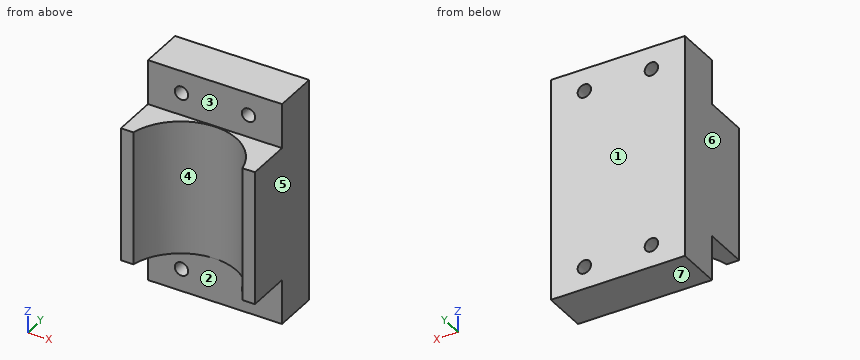
from build123d import *

# Parameters (mm, degrees)
F0_W     = 30
F0_H     = 50
F1_DEPTH = 10
F2_R     = 1.5
F3_DEPTH = 10.001
F4_W     = 30
F4_H     = 30
F5_DEPTH = 10
F6_R     = 12.5
F7_DEPTH = 25.001
F8_DEPTH = 25.001


with BuildPart() as f1:
    # F0 (on Front) → F1 (new body)
    with BuildSketch(Plane.XZ):
        Rectangle(F0_W, F0_H)
    extrude(amount=F1_DEPTH)

    # F2 (on face) → F3 (cut, through all)
    with BuildSketch(Plane.XZ.offset(10)):
        with Locations((7.5, -20)):
            Circle(F2_R)
        with Locations((-7.5, -20)):
            Circle(F2_R)
        with Locations((7.5, 20)):
            Circle(F2_R)
        with Locations((-7.5, 20)):
            Circle(F2_R)
    extrude(amount=-F3_DEPTH, mode=Mode.SUBTRACT)

    # F4 (on face) → F5 (join)
    with BuildSketch(Plane.XZ.offset(10)):
        Rectangle(F4_W, F4_H)
    extrude(amount=F5_DEPTH)

    # F6 (on Top) → F7 (cut, through all)
    with BuildSketch(Plane.XY):
        with Locations((0, -22.66825)):
            Circle(F6_R)
    extrude(amount=-F7_DEPTH, mode=Mode.SUBTRACT)

    # F6 (on Top) → F8 (cut, through all)
    with BuildSketch(Plane.XY):
        with Locations((0, -22.66825)):
            Circle(F6_R)
    extrude(amount=F8_DEPTH, mode=Mode.SUBTRACT)


solid = f1.part
Geometry: final body of the model. Coordinates: model frame, mm. Face numbers are marked on the shaded views. A direction names the side the tool comes from. Coordinates: 2 decimals unless noted, no trailing zeros. Loops run counter-clockwise (first coordinate to the right, second up) from the corner with the lowest first, then second, coordinate; pieces in that order, holes last. Notation, with made-up numbers: (-0.5, 12.5) - (19.5, 12.5) arc R15 cw to (19.5, 32.5) - close; hole circle Ø7 at (-33.5, 61). An arc over 180 degrees is marked (long way). Put each result on its own line as item: value. Start each with the question number.
Q1. Set-up query: the marked faces 1, 2 and 3. Return all of +Z, -Z, +X, -X, +Y, -Y with unobstructed straight access to the full face (end or side cutting, diameter ignored); none if empty.
Q2. Cut plane D-D, the plane y = -16.5. Return loops of the section in (x, z), and give its area (3 significant figures).
Q3. Cut plane A-A, the plane z = -20. Return loops of the section in (x, y).
Q4. Cut plane B-B, the plane y = -6.25. Return loops of the section in (x, z), and give its area (3 significant figures).
Q5. Pull-direction query (X, two-part tool) for the marked faces 4, 5, 6 and 7; classes: released by +X, released by -X, zero draft, split by the parting line, or undercut.
Q6. Cut plane C-C, the plane x = 7.5. Return loops of the section in (y, z).
Q7. Pin query (flat end, axial travel): pin 1 Ø1.8 at (x, z) = (-7.5, -20) entering from -Y; pin 2 Ø6 at (x, y) = (11, -15) entering from -Z; pin 3 Ø3 at (x, z) = (-3.5, 20.5) entering from -Y; pin 4 Ø6 at (x, z) = (0, -8) entering from -Y. Return the tip coordinate at first contact, or that it passes through.
Q8. Line query: line 1 (Z direction, x = 7.5, y = -3); line 2 (Y direction, x = 4.75, z = -19); line 3 (Z direction, x = -10, y = -11.5). Output: solid intervals per line, ascending.
Filled sheet:
1. face 1: +Z, -Z, +X, -X, +Y
1. face 2: -Z, +X, -X, -Y
1. face 3: +Z, +X, -X, -Y
2. outline: (-15, -15) - (-10.87, -15) - (-10.87, 15) - (-15, 15) - close; (10.87, -15) - (15, -15) - (15, 15) - (10.87, 15) - close
2. area: 248 mm²
3. outline: (-15, -10) - (-9, -10) - (-9, 0) - (-15, 0) - close; (-6, -10) - (6, -10) - (6, 0) - (-6, 0) - close; (9, -10) - (15, -10) - (15, 0) - (9, 0) - close
4. outline: (-15, -25) - (15, -25) - (15, 25) - (-15, 25) - close; hole circle Ø3 at (-7.5, -20); hole circle Ø3 at (-7.5, 20); hole circle Ø3 at (7.5, -20); hole circle Ø3 at (7.5, 20)
4. area: 1,470 mm²
5. face 4: undercut
5. face 5: released by +X
5. face 6: released by -X
5. face 7: zero draft
6. outline: (-12.67, -15) - (-10, -15) - (-10, -18.5) - (0, -18.5) - (0, 18.5) - (-10, 18.5) - (-10, 15) - (-12.67, 15) - close; (-10, -25) - (0, -25) - (0, -21.5) - (-10, -21.5) - close; (-10, 21.5) - (0, 21.5) - (0, 25) - (-10, 25) - close
7. pin 1: through
7. pin 2: z = -15
7. pin 3: y = -10
7. pin 4: y = -10.53
8. line 1: -25 to -21.5, -18.5 to 18.5, 21.5 to 25
8. line 2: -10 to 0
8. line 3: -15 to 15
